CAD build for the part. Positions are in the model's coordinates, mm. Face numbers are marked on the shaded views. A direction names the side the tool comes from. Coordinates: 2 decimals unless noted, no trailing zeros. Loops run counter-clockwise (first coordinate to the right, second up) from the corner with the lowest first, then second, coordinate; pieces in that order, holes last. Notation, with made-up numbers: (14, 66) -> (68, 66) arc R16 ccw to (68, 76) -> close; hole circle Ø5 at (89.5, -8.5). An arc over 180 degrees is marked (long way). Write each question's results on one line, items separated by ' | '.
```python
from build123d import *

# Parameters (mm, degrees)
F1_DEPTH = 28
F2_R     = 1.5
F3_DEPTH = 5
F4_R     = 1.5
F5_DEPTH = 3


with BuildPart() as f1:
    # F0 (on Top) → F1 (new body)
    with BuildSketch(Plane.XY):
        Polygon((3.5371081789, -0.8478594996), (2.5028219549, 2.639295789), (-1.0342862239, 3.4871552886), (-3.5371081789, 0.8478594996), (-2.5028219549, -2.639295789), (1.0342862239, -3.4871552886), align=None)
    extrude(amount=F1_DEPTH)

    # F2 (on face) → F3 (join)
    with BuildSketch(Plane.XY.offset(28)):
        Circle(F2_R)
    extrude(amount=F3_DEPTH)

    # F4 (on face) → F5 (join)
    with BuildSketch(Plane(origin=(0, 0, 0), x_dir=(1, 0, 0), z_dir=(0, 0, -1))):
        Circle(F4_R)
    extrude(amount=F5_DEPTH)


solid = f1.part
```
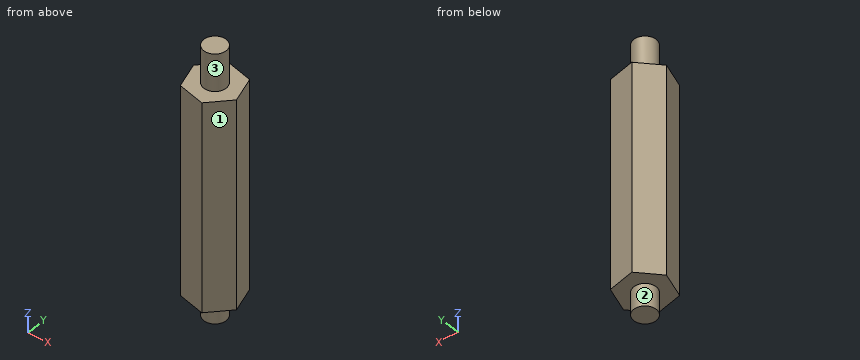
Q1. Cut at D-D on x = -2. Write the cut outline in (y, z), and give its area (3 significant figures).
Results are:
outline: (-2.76, 0) -> (2.47, 0) -> (2.47, 28) -> (-2.76, 28) -> close | area: 146 mm^2
Q2. Wall check: L1, parallel to Z at x = 2, y = -2; L2, parallel to Y at x = -2.25, z = 26; L3, parallel to X at y = -1, z = 7. Give the ranges that are in metal, low to high. Write a range as from..to.
Results are:
L1: 0..28 | L2: -2.7..2.21 | L3: -2.99..3.39
Q3. Cut at B-B on z = 7. Write the cut outline in (x, y), and give its area (3 significant figures).
Results are:
outline: (-3.54, 0.85) -> (-2.5, -2.64) -> (1.03, -3.49) -> (3.54, -0.85) -> (2.5, 2.64) -> (-1.03, 3.49) -> close | area: 34.4 mm^2
Q4. Cut at A-A on x = 0.5. Write the cut outline in (y, z), and give its area (3 significant figures).
Results are:
outline: (-3.36, 0) -> (-1.41, 0) -> (-1.41, -3) -> (1.41, -3) -> (1.41, 0) -> (3.12, 0) -> (3.12, 28) -> (1.41, 28) -> (1.41, 33) -> (-1.41, 33) -> (-1.41, 28) -> (-3.36, 28) -> close | area: 204 mm^2
Q5. Cut at C-C on y = 0.5. Write the cut outline in (x, z), and give its area (3 significant figures).
Results are:
outline: (-3.43, 0) -> (-1.41, 0) -> (-1.41, -3) -> (1.41, -3) -> (1.41, 0) -> (3.14, 0) -> (3.14, 28) -> (1.41, 28) -> (1.41, 33) -> (-1.41, 33) -> (-1.41, 28) -> (-3.43, 28) -> close | area: 207 mm^2
Q6. Which spindle directions (+Z, -Z, +X, -X, +Y, -Y) get a long thin tool onto all of the face, cutting with end or side? Do the marked faces 1, 2 and 3. Say none if no direction does.
Results are:
face 1: +Z, -Z, +X, -Y | face 2: -Z | face 3: +Z
Q7. Drop flat-ended pins along their axis: pin 1 (1.5 mm diameter, centred on x = -2, z = 20, fed in from -Y); pin 2 (1.5 mm diameter, centred on x = 2, y = 2.5, fed in from +Z). Give the stop position or say it passes through.
Results are:
pin 1: y = -2.94 | pin 2: z = 28
